Can you work these out from the model? Positions are in its coordinate system, mm. Give positions to 0.01 mm unless a question says otherwise; leave off trailing zeros. Order: outer loops, then holes, each group sorted by start corner. A loop starts at its lowest first (then second) coordinate and runs counter-clockwise, first axis right, second up. Notation, with made-up numbers: M -34,-11 L -29,-11 A10 cw -29,-4 Z; hole C 11,34 d6. An arc over 180 degrees is marked long. One line per question, with ' | ' between items. Start each with the question number.
1) I'm going to push a flat-ended pin straight in: pin 1 Ø4 at (x, y) = (95, 0) entering from +Z (3 decimals). Where does the tip first touch, or does it pass through?
2) If we section it at A-A, the plane x = 259: Please give me the cut outline in (y, z).
3) Please list where these lines run through material, in increasing order: line 1 along Y through (x, z) = (75.5, -5); line 2 along Z through (x, y) = (140, -7.05). Write a range as [from, to].
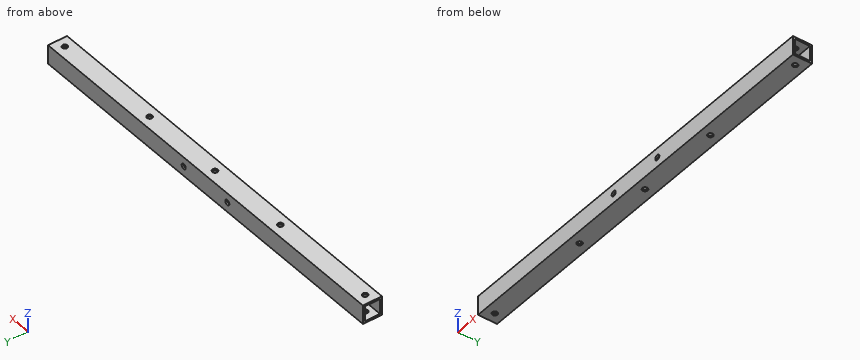
```python
from build123d import *

# Parameters (mm, degrees)
SKETCH_1_W          = 15
SKETCH_1_H          = 15
SKETCH_1_W_2        = 12
SKETCH_1_H_2        = 12
EXTRUDE_1_DEPTH     = 325
SKETCH_2_R          = 2.1
CUT_EXTRUDE_1_DEPTH = 326.432404656
SKETCH_3_R          = 2.1
CUT_EXTRUDE_2_DEPTH = 326.432404656
SKETCH_4_R          = 2.1
CUT_EXTRUDE_3_DEPTH = 326.432404656


with BuildPart() as part:
    # ｽｹｯﾁ1 → 押し出し-薄板1 (new body)
    with BuildSketch(Plane(origin=(0, 0, 0), x_dir=(0, 0, -1), z_dir=(1, 0, 0))):
        Rectangle(SKETCH_1_W, SKETCH_1_H)
        Rectangle(SKETCH_1_W_2, SKETCH_1_H_2, mode=Mode.SUBTRACT)
    extrude(amount=EXTRUDE_1_DEPTH)

    # ｽｹｯﾁ2 → ｶｯﾄ - 押し出し1 (cut, through all)
    with BuildSketch(Plane.XY.offset(7.5)):
        with Locations((7.5, 0)):
            Circle(SKETCH_2_R)
        with Locations(Location((317.5, 0, 0), (0, 0, 90))):
            Circle(SKETCH_2_R)
    extrude(amount=-CUT_EXTRUDE_1_DEPTH, mode=Mode.SUBTRACT)

    # ｽｹｯﾁ3 → ｶｯﾄ - 押し出し2 (cut, through all)
    with BuildSketch(Plane.XY.offset(7.5)):
        with Locations((95, 0)):
            Circle(SKETCH_3_R)
        with Locations(Location((230, 0, 0), (0, 0, 90))):
            Circle(SKETCH_3_R)
        with Locations((162.5, 0)):
            Circle(SKETCH_3_R)
    extrude(amount=-CUT_EXTRUDE_2_DEPTH, mode=Mode.SUBTRACT)

    # ｽｹｯﾁ4 → ｶｯﾄ - 押し出し3 (cut, through all)
    with BuildSketch(Plane(origin=(0, 7.5, 0), x_dir=(1, 0, 0), z_dir=(0, 1, 0))):
        with Locations(Location((140, 0, 0), (0, 0, 270))):
            Circle(SKETCH_4_R)
        with Locations(Location((185, 0, 0), (0, 0, 270))):
            Circle(SKETCH_4_R)
    extrude(amount=-CUT_EXTRUDE_3_DEPTH, mode=Mode.SUBTRACT)


solid = part.part
```
Results found:
1) pin 1: passes through
2) outline: M -7.5,-7.5 L 7.5,-7.5 L 7.5,7.5 L -7.5,7.5 Z; hole M -6,-6 L 6,-6 L 6,6 L -6,6 Z
3) line 1: y = [-7.5, -6], [6, 7.5] | line 2: z = [-7.5, -2.1], [2.1, 7.5]
